Input: part model. Units: mm. Frame: model coordinates. Give positions to 0.01 mm unless a question says otherwise; leave off trailing zeros. Write each loop counter-clockwise with the first axis right and the second up, starting at its lowest first coordinate (ties: lowest second). Pieces come first, ordered by that corner, then holes. Notation, with made-up numbers: (12.5, -32.5) -> (16.5, -32.5) arc R10 cw to (16.5, -15.5) -> close; hole circle Ø6 at (74.25, 36.5). An arc over 180 degrees is marked (long way). Answer as a JSON object with one key per item and string values. Group by question number.
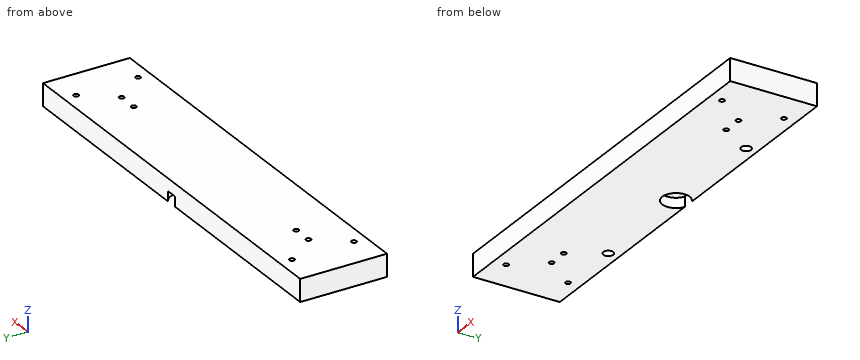
from build123d import *

# Parameters (mm, degrees)
CYLINDER005_R     = 11
CYLINDER005_DEPTH = 8
CYLINDER004_R     = 4
CYLINDER004_DEPTH = 10
CYLINDER002_R     = 2
CYLINDER002_DEPTH = 25
CYLINDER001_R     = 2
CYLINDER001_DEPTH = 25
CYLINDER_R        = 2
CYLINDER_DEPTH    = 25
CYLINDER003_R     = 2
CYLINDER003_DEPTH = 25
BOX_W             = 168
BOX_H             = 70
BOX_DEPTH         = 18


with BuildPart() as cilindro005:
    # Cylinder005 → Cylinder005 (new body)
    with BuildSketch(Plane(origin=(168, 60, 0), x_dir=(1, 0, 0), z_dir=(0, 0, 1))):
        Circle(CYLINDER005_R)
    extrude(amount=CYLINDER005_DEPTH)


with BuildPart() as cilindro004:
    # Cylinder004 → Cylinder004 (new body)
    with BuildSketch(Plane(origin=(78, 61, 0), x_dir=(1, 0, 0), z_dir=(0, 0, 1))):
        Circle(CYLINDER004_R)
    extrude(amount=CYLINDER004_DEPTH)


with BuildPart() as cilindro002:
    # Cylinder002 → Cylinder002 (new body)
    with BuildSketch(Plane(origin=(46, 35, 0), x_dir=(1, 0, 0), z_dir=(0, 0, 1))):
        Circle(CYLINDER002_R)
    extrude(amount=CYLINDER002_DEPTH)


with BuildPart() as cilindro001:
    # Cylinder001 → Cylinder001 (new body)
    with BuildSketch(Plane(origin=(27, 60, 0), x_dir=(1, 0, 0), z_dir=(0, 0, 1))):
        Circle(CYLINDER001_R)
    extrude(amount=CYLINDER001_DEPTH)


with BuildPart() as cilindro:
    # Cylinder → Cylinder (new body)
    with BuildSketch(Plane(origin=(27, 10, 0), x_dir=(1, 0, 0), z_dir=(0, 0, 1))):
        Circle(CYLINDER_R)
    extrude(amount=CYLINDER_DEPTH)


with BuildPart() as fusion:
    # Cylinder003 → Cylinder003 (new body)
    with BuildSketch(Plane(origin=(62, 35, 0), x_dir=(1, 0, 0), z_dir=(0, 0, 1))):
        Circle(CYLINDER003_R)
    extrude(amount=CYLINDER003_DEPTH)

    # Fusion: union Cilindro004, Cilindro002, Cilindro001, Cilindro
    add(cilindro004.part)
    add(cilindro002.part)
    add(cilindro001.part)
    add(cilindro.part)


with BuildPart() as cut:
    # Box → Box (new body)
    with BuildSketch(Plane.XY):
        with Locations((84, 35)):
            Rectangle(BOX_W, BOX_H)
    extrude(amount=BOX_DEPTH)

    # Cut: cut Fusion
    add(fusion.part, mode=Mode.SUBTRACT)


with BuildPart() as cut001:
    # mirror: instance of Cut
    add(cut.part.mirror(Plane(origin=(168, 0, 0), x_dir=(0, -1, 0), z_dir=(1, 0, 0))))

    # Fusion001: union Cut
    add(cut.part)

    # Cut001: cut Cilindro005
    add(cilindro005.part, mode=Mode.SUBTRACT)


solid = cut001.part
1. Contact query for flat-ended pins moving along their axis: pin 1 Ø3 at (x, y) = (138.5, 39.5) entering from -Z; pin 2 Ø20 at (x, y) = (168, 60) entering from -Z; pin 3 Ø4 at (x, y) = (258, 60) entering from -Z. Output: stop coordinate, or through.
2. Section B-B (z = 4.25). State how many separate pieces and enclosed holes the cut face has, plus the area to 3 significant figures.
3. Line query: line 1 (X direction, y = 60, z = 10.25); line 2 (Y direction, x = 27, z = 6.75); line 3 (X direction, y = 34.5, z = 4). Output: solid intervals per line, ascending.
4. Section A-A (x = 258). Return the cut outline in (y, z), plus the area to 3 significant figures.
5. Section C-C (x = 168). Return the cut outline in (y, z), plus the area to 3 significant figures.
Working result:
{
 "1": {"pin 1": "stops at z = 0", "pin 2": "stops at z = 8", "pin 3": "stops at z = 10"},
 "2": {"separate pieces": "1", "enclosed holes": "10", "area": "22,900 mm^2"},
 "3": {"line 1": "x = 0 to 25, 29 to 307, 311 to 336", "line 2": "y = 0 to 8, 12 to 58, 62 to 70", "line 3": "x = 0 to 44.06, 47.94 to 60.06, 63.94 to 272.06, 275.94 to 288.06, 291.94 to 336"},
 "4": {"outline": "(0, 0) -> (57, 0) -> (57, 10) -> (65, 10) -> (65, 0) -> (70, 0) -> (70, 18) -> (0, 18) -> close", "area": "1,180 mm^2"},
 "5": {"outline": "(0, 0) -> (49, 0) -> (49, 8) -> (70, 8) -> (70, 18) -> (0, 18) -> close", "area": "1,090 mm^2"}
}
